For this review, take the finished solid that the model builds, in its own axes (mm). Face numbers are marked on the shaded views. Round coordinates to 2 decimals unless told otherwise and drop trailing zeros. Write each loop counter-clockwise with the first axis right and the second up, starting at its lowest first coordinate (ties: lowest second). Pieces come first, ordered by that corner, then holes. Notation, with made-up numbers: (-34, 72.5) -> (-29, 72.5) arc R18 cw to (-29, 84.5) -> close; hole circle Ø5 at (18.25, 52). An arc over 180 degrees is marked (long way). Answer as CSV lines item,"result". Start each with the question number.
Item 1: Take a section at B-B on y = -5. Give the boundary of the cut face in (x, z).
Item 2: Take a section at A-A on x = 0. Give the boundary of the cut face in (y, z).
Item 3: Wall thickness on probe 1 along Z at (x, y) = (0, -7.5); probe 2 along X at (y, z) = (-5, -4); probe 3 along Z at (x, y) = (0.75, -14): over which ranges is each line inside the solid? List them lowest first. Write a range as from..to.
Item 4: For pin 1 Ø3 at (x, y) = (0, -20) entering from -Z; pin 2 Ø1.5 at (x, y) = (0, -5) entering from -Z; pin 3 Ø2 at (x, y) = (4, -6.5) entering from -Z; pin 4 Ø2 at (y, z) = (-21.5, -1.5) entering from -X, all flat-tipped, find the tip position at first contact; note any pin that passes through.
Item 5: Mouldability with a two-part tool opening along Y and no side actions: class the marked faces 1, 2, 3 and 4 as +Y half, -Y half, draft (parallel to the pull), parting line (faces both ways), or undercut.
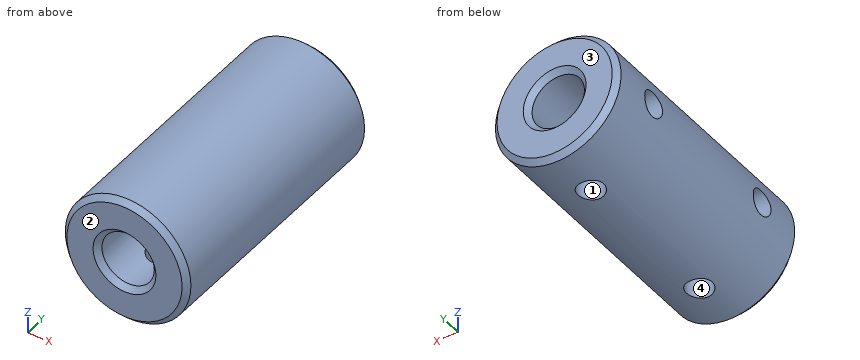
```python
from build123d import *

# Parameters (mm, degrees)
F0_R     = 6
F0_R_2   = 2.5
F1_DEPTH = 25
F2_R     = 1.2295
F3_DEPTH = 25
F4_R     = 1.2295
F5_DEPTH = 25
F6_SIZE  = 0.5


with BuildPart() as f1:
    # F0 (on Front) → F1 (new body)
    with BuildSketch(Plane.XZ):
        Circle(F0_R)
        Circle(F0_R_2, mode=Mode.SUBTRACT)
    extrude(amount=F1_DEPTH)

    # F2 (on Top) → F3 (cut)
    with BuildSketch(Plane.XY):
        with Locations((0, -5)):
            Circle(F2_R)
        with Locations((0, -20)):
            Circle(F2_R)
    extrude(amount=-F3_DEPTH, mode=Mode.SUBTRACT)

    # F4 (on Right) → F5 (cut)
    with BuildSketch(Plane.YZ):
        with Locations((-5, 0)):
            Circle(F4_R)
        with Locations((-20, 0)):
            Circle(F4_R)
    extrude(amount=-F5_DEPTH, mode=Mode.SUBTRACT)

    # F6
    f6_edges = [f1.edges().sort_by_distance(p)[0] for p in [
        (-6, -25, 0),
        (-2.5, -25, 0),
        (-6, 0, 0),
        (-2.5, 0, 0),
    ]]
    chamfer(f6_edges, length=F6_SIZE)


solid = f1.part
```
Output values:
1,outline,"(-5.87, -1.23) arc R6 ccw to (-1.23, -5.87) -> (-1.23, -2.18) arc R2.5 cw to (-2.18, -1.23) -> close; (-5.87, 1.23) -> (-2.18, 1.23) arc R2.5 cw (long way) to (1.23, -2.18) -> (1.23, -5.87) arc R6 ccw (long way) to start"
2,outline,"(-25, -5.5) -> (-24.5, -6) -> (-21.23, -6) -> (-21.23, -2.5) -> (-24.5, -2.5) -> (-25, -3) -> close; (-25, 3) -> (-24.5, 2.5) -> (-0.5, 2.5) -> (0, 3) -> (0, 5.5) -> (-0.5, 6) -> (-24.5, 6) -> (-25, 5.5) -> close; (-18.77, -6) -> (-6.23, -6) -> (-6.23, -2.5) -> (-18.77, -2.5) -> close; (-3.77, -6) -> (-0.5, -6) -> (0, -5.5) -> (0, -3) -> (-0.5, -2.5) -> (-3.77, -2.5) -> close"
3,probe 1,"z = -6..-2.5, 2.5..6"
3,probe 2,"x = -4.47..-1.23, 1.23..4.47"
3,probe 3,"z = -5.95..-2.38, 2.38..5.95"
4,pin 1,"stops at z = -6"
4,pin 2,"stops at z = 2.38"
4,pin 3,"stops at z = -5.2"
4,pin 4,"stops at x = -5.98"
5,face 1,"undercut"
5,face 2,"-Y half"
5,face 3,"+Y half"
5,face 4,"undercut"
